Verification items for the finished model (mm, model axes). Face numbers are marked on the shaded views. A direction names the side the tool comes from. Give positions to 0.01 mm unless a question says otherwise; leave off trailing zeros. Order: outer loops, then holes, each group sorted by start corner. A loop starts at its lowest first (then second) coordinate and runs counter-clockwise, first axis right, second up.
from build123d import *

# Parameters (mm, degrees)
SKETCH_1_R          = 3
SKETCH_1_R_2        = 7.5
EXTRUDE_2_DEPTH     = 45
SKETCH_3_W          = 65
SKETCH_3_H          = 65
CUT_EXTRUDE_1_DEPTH = 35
FILLET_1_R          = 3


with BuildPart() as part:
    # ｽｹｯﾁ1 → ﾎﾞｽ - 押し出し2 (new body)
    with BuildSketch(Plane.XY):
        with BuildLine():
            Line((0, 0), (60.482195673, 0))
            Line((60.482195673, 0), (96.609428685, 53.858775707))
            ThreePointArc((96.609428685, 53.858775707), (97.646876294, 74.412106941), (80, 85))
            Line((80, 85), (49.635590302, 85))
            ThreePointArc((49.635590302, 85), (42.822728652, 86.91697026), (38.00913265, 92.105337282))
            ThreePointArc((38.00913265, 92.105337282), (31.226913615, 96.915979081), (23.397413698, 94.116032547))
            Line((23.397413698, 94.116032547), (0, 68.857265202))
            Line((0, 68.857265202), (0, 0))
        make_face()
        with Locations(Location((30, 88, 0), (0, 0, 180))):
            Circle(SKETCH_1_R, mode=Mode.SUBTRACT)
        with Locations(Location((80, 65, 0), (0, 0, 180))):
            Circle(SKETCH_1_R_2, mode=Mode.SUBTRACT)
    extrude(amount=EXTRUDE_2_DEPTH)

    # ｽｹｯﾁ3 → ｶｯﾄ - 押し出し1 (cut)
    with BuildSketch(Plane.XY.offset(45)):
        with Locations((32.5, 32.5)):
            Rectangle(SKETCH_3_W, SKETCH_3_H)
    extrude(amount=-CUT_EXTRUDE_1_DEPTH, mode=Mode.SUBTRACT)

    # ﾌｨﾚｯﾄ1
    fillet_1_edges = [part.edges().sort_by_distance(p)[0] for p in [
        (0, 0, 5),
    ]]
    fillet(fillet_1_edges, radius=FILLET_1_R)


solid = part.part
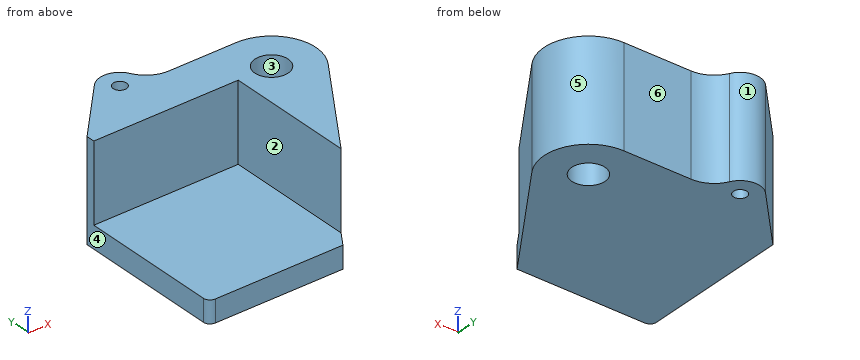
(1) Section check D-D, the plane x = 54. Enter the section's corners in (y, z), then the cut area to 3 significant figures.
Solved:
outline: (0, 0) - (85, 0) - (85, 45) - (65, 45) - (65, 10) - (0, 10) - close
area: 1,550 mm2
(2) Scan lines: line 1 (Y direction, x = 30, z = 17.5); line 2 (Z direction, x = 13, y = 62.5); line 3 (X direction, y = 88, z = 28). Record each from-to range of solid material in increasing order.
Solved:
line 1: y = 65 to 85, 91 to 97
line 2: z = 0 to 10
line 3: x = 17.73 to 27, 33 to 41.31
(3) Section check B-B, the plane z = 19. Enter the section's corners in (x, y).
Solved:
outline: (0, 65) - (65, 65) - (65, 6.74) - (96.61, 53.86) arc R20 ccw to (80, 85) - (49.64, 85) arc R13.06 cw to (38.01, 92.11) arc R9 ccw to (23.4, 94.12) - (0, 68.86) - close; hole circle Ø6 at (30, 88); hole circle Ø15 at (80, 65)
(4) Set-up check for the marked faces 1 and 2: record each of +Z, -Z, +X, -X, +Y, -Y from which the full face is reachable in a straight line by a thin tool's end or side.
Solved:
face 1: +Z, -Z, +Y
face 2: +Z, -X, -Y
(5) Release check for a two-part mould opening along Y. For the marked faces 3, 4, 5 and 6 record: pulls with the +Y half, pulls with the -Y half, needs draft (parallel to the pull), parting line crosses it, or undercut.
Solved:
face 3: undercut
face 4: needs draft
face 5: parting line crosses it
face 6: pulls with the +Y half
(6) Section check C-C, the plane y = 88. Enter the section's corners in (x, z).
Solved:
outline: (17.73, 0) - (27, 0) - (27, 45) - (17.73, 45) - close; (33, 0) - (41.31, 0) - (41.31, 45) - (33, 45) - close
(7) Section check A-A, the plane x = 30. Enter the section's corners in (y, z).
Solved:
outline: (0, 0) - (85, 0) - (85, 45) - (65, 45) - (65, 10) - (0, 10) - close; (91, 0) - (97, 0) - (97, 45) - (91, 45) - close
(8) Go/stop test with flat-tipped pins: pin 1 (2 mm diameter, centred on x = 13, y = 59, fed in from +Z); pin 2 (1.5 mm diameter, centred on y = 60, z = 30, fed in from -X); pin 3 (2 mm diameter, centred on x = 88.5, z = 39, fed in from -Y); pin 4 (9 mm diameter, centred on x = 80, y = 65, fed in from -Z). Record where each tip stops, or that it passes through.
Solved:
pin 1: stops at z = 10
pin 2: stops at x = 65
pin 3: stops at y = 40.28
pin 4: passes through
